Source: CAD feature listing. Evaluate the final solid. Frame: model axes, mm. Face numbers are marked on the shaded views. A direction names the side the tool comes from. Give positions to 0.01 mm unless a question says otherwise; leave off trailing zeros. Order: outer loops, then holes, each group sorted by start corner. A loop starts at its lowest first (then second) coordinate and runs counter-clockwise, first axis right, second up. Notation, with made-up numbers: M 59.25,55.5 L 67.25,55.5 A17 cw 67.25,85.5 Z; hole C 32.25,85 d2. An arc over 180 degrees is marked long. One line per question, with ' | ' between items. Start each with the question number.
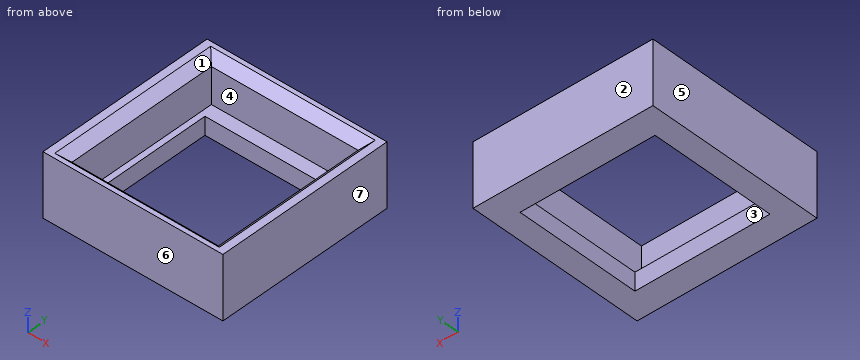
from build123d import *

# Parameters (mm, degrees)
SKETCH_W      = 20
SKETCH_H      = 20
SKETCH_W_2    = 15
SKETCH_H_2    = 14
PAD_DEPTH     = 2
SKETCH001_W   = 20
SKETCH001_H   = 20
SKETCH001_W_2 = 16.3
SKETCH001_H_2 = 17
PAD001_DEPTH  = 5
CHAMFER_SIZE  = 1


with BuildPart() as part:
    # Sketch → Pad (new body)
    with BuildSketch(Plane.XY):
        Rectangle(SKETCH_W, SKETCH_H)
        Rectangle(SKETCH_W_2, SKETCH_H_2, mode=Mode.SUBTRACT)
    extrude(amount=PAD_DEPTH)

    # Sketch001 (on Face10 of Pad) → Pad001 (join)
    with BuildSketch(Plane.XY.offset(2)):
        Rectangle(SKETCH001_W, SKETCH001_H)
        Rectangle(SKETCH001_W_2, SKETCH001_H_2, mode=Mode.SUBTRACT)
    extrude(amount=PAD001_DEPTH)

    # Chamfer
    chamfer_edges = [part.edges().sort_by_distance(p)[0] for p in [
        (0, 8.5, 7),
        (-8.15, 0, 7),
        (0, -8.5, 7),
        (8.15, 0, 7),
    ]]
    chamfer(chamfer_edges, length=CHAMFER_SIZE)


solid = part.part
Item 1: Reachability of the marked faces 1, 2 and 3 from +Z, -Z, +X, -X, +Y, -Y: full face, straight path, thin tool, end or side. Return the list, or none.
Item 2: Cut plane A-A on z = 2.5. Return the cut outline in (x, y).
Item 3: Cut plane D-D on y = -7.25. Return the cut outline in (x, z), and give its area (3 significant figures).
Item 4: Line query: line 1 (Y direction, x = -4.75, z = 3.5); line 2 (Y direction, x = -7.25, z = 0.5); line 3 (X direction, y = 6.5, z = 3.5). Output: solid intervals per line, ascending.
Item 5: Cut plane B-B on x = 5.25. Return the cut outline in (y, z).
Item 6: Mould query, pull axis X, two halves, no side actions, for the marked faces 4, 5, 6 and 7. Classes: pulls with the +X half, pulls with the -X half, needs draft (parallel to the pull), parting line crosses it, or undercut.
Item 7: Pin query (flat end, axial travel): pin 1 Ø4 at (x, y) = (-5, 0) entering from +Z; pin 2 Ø5 at (x, y) = (7.5, 0.5) entering from -Z. Return the tip coordinate at first contact, or that it passes through.
Item 8: Cut plane C-C on y = -2.5. Return the cut outline in (x, z), and give its area (3 significant figures).
Results are:
1) face 1: +Z | face 2: +Z, -Z, +X, -X, +Y | face 3: +Z, -Z
2) outline: M -10,-10 L 10,-10 L 10,10 L -10,10 Z; hole M -8.15,-8.5 L 8.15,-8.5 L 8.15,8.5 L -8.15,8.5 Z
3) outline: M -10,0 L 10,0 L 10,7 L 9.15,7 L 8.15,6 L 8.15,2 L -8.15,2 L -8.15,6 L -9.15,7 L -10,7 Z | area: 57.5 mm2
4) line 1: y = -10 to -8.5, 8.5 to 10 | line 2: y = -10 to -7, 7 to 10 | line 3: x = -10 to -8.15, 8.15 to 10
5) outline: M -10,0 L -7,0 L -7,2 L -8.5,2 L -8.5,6 L -9.5,7 L -10,7 Z; M 7,0 L 10,0 L 10,7 L 9.5,7 L 8.5,6 L 8.5,2 L 7,2 Z
6) face 4: undercut | face 5: pulls with the -X half | face 6: needs draft | face 7: pulls with the +X half
7) pin 1: passes through | pin 2: stops at z = 0
8) outline: M -10,0 L -7.5,0 L -7.5,2 L -8.15,2 L -8.15,6 L -9.15,7 L -10,7 Z; M 7.5,0 L 10,0 L 10,7 L 9.15,7 L 8.15,6 L 8.15,2 L 7.5,2 Z | area: 27.5 mm2
